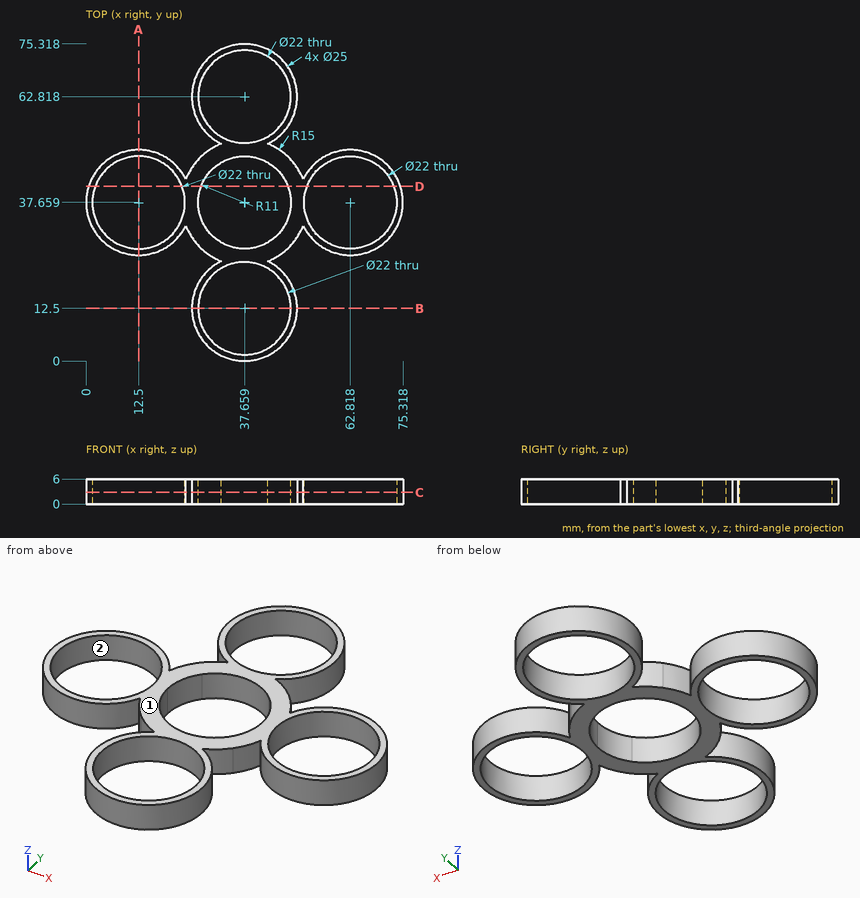
Study the drawing (mm; zero at the part's minimum x, y, z) and answer. Give positions to 0.01 mm unless a question says otherwise; leave off trailing zeros. Loops run counter-clockwise (first coordinate to the right, second up) from the corner with the lowest first, then second, coordinate; pieces in that order, holes last. Notation, with made-up numbers: (5, 87.5) - (40, 87.5) arc R23 cw to (40, 122.5) - close; hole circle Ø9 at (-20.5, 59.5). An arc over 180 degrees is marked (long way). Return JSON: item names as keys, results as strings. Group by question number.
1. Find section C-C (z = 2.85). Write down the section's boundary in (x, y) (1 decimal).
2. Determine the mould class of the marked faces 1 and 2 for opening direction Y: pulls with the +Y half, pulls with the -Y half, needs draft (parallel to the pull), parting line crosses it, or undercut.
3. Straight lines are drawn through the part: line 1 (Y direction, x = 63, z = 5.8); line 2 (X direction, y = 34.5, z = 0.9) (1 decimal); line 3 (X direction, y = 27.5, z = 0.9) (1 decimal). For each, find the intervals that lie inside material, in ascending order. Write a range as [from, to].
4. Find section A-A (x = 12.5). Write down the section's boundary in (y, z).
5. Find section D-D (y = 41.5). Write down the section's boundary in (x, z) (1 decimal).
6. Given pin 1 Ø3 at (y, z) = (18.5, 5) entering from +X; pin 2 Ø1 at (x, z) = (51, 3) entering from +Y; pin 3 Ø1.5 at (x, z) = (67.5, 4) entering from -Y, each flat-ended and moving along its own axis, determine where each tip first touches the part or whether it passes through.
Verdict:
{
 "1": {"outline": "(23.7, 32.1) arc R15 ccw to (32.1, 23.7) arc R12.5 ccw (long way) to (43.2, 23.7) arc R15 ccw to (51.6, 32.1) arc R12.5 ccw (long way) to (51.6, 43.2) arc R15 ccw to (43.2, 51.6) arc R12.5 ccw (long way) to (32.1, 51.6) arc R15 ccw to (23.7, 43.2) arc R12.5 ccw (long way) to start; hole circle Ø22 at (12.5, 37.7); hole circle Ø22 at (37.7, 12.5); hole circle Ø22 at (37.7, 62.8); hole (29.9, 29.9) arc R11 ccw to (45.4, 29.9) arc R11 ccw to (45.4, 45.4) arc R11 ccw to (29.9, 45.4) arc R11 ccw to start; hole circle Ø22 at (62.8, 37.7)"},
 "2": {"face 1": "needs draft", "face 2": "undercut"},
 "3": {"line 1": "y = [25.16, 26.66], [48.66, 50.16]", "line 2": "x = [0.4, 2], [23, 27.1], [48.2, 52.3], [73.4, 74.9]", "line 3": "x = [5.2, 8.3], [16.7, 19.8], [26.6, 33.4], [41.9, 48.7], [55.5, 58.6], [67, 70.1]"},
 "4": {"outline": "(25.16, 0) - (26.66, 0) - (26.66, 6) - (25.16, 6) - close; (48.66, 0) - (50.16, 0) - (50.16, 6) - (48.66, 6) - close"},
 "5": {"outline": "(0.6, 0) - (2.2, 0) - (2.2, 6) - (0.6, 6) - close; (22.8, 0) - (27.4, 0) - (27.4, 6) - (22.8, 6) - close; (48, 0) - (52.5, 0) - (52.5, 6) - (48, 6) - close; (73.1, 0) - (74.7, 0) - (74.7, 6) - (73.1, 6) - close"},
 "6": {"pin 1": "stops at x = 49.32", "pin 2": "stops at y = 45.41", "pin 3": "stops at y = 25.79"}
}
